Work out the finished part from the listing and answer in its coordinate system (mm). A direction names the side the tool comes from. Round coordinates to 2 decimals unless told otherwise and drop trailing zeros. Order: outer loops, then holes, each group sorted by start corner. A loop starts at its lowest first (then second) coordinate and runs counter-clockwise, first axis right, second up. Notation, with made-up numbers: (34.25, -20) -> (89.25, -20) arc R13 ccw to (89.25, -8) -> close; hole circle Ø3 at (5.25, 62.25). An arc over 180 degrees is marked (long way). Use a Markdown table: item, result. Add a question column.
Item 1: A cutting plane is placed at A-A, the plane z = 5.5. Determine the outline of the cut face in (x, y), plus the area to 3 significant figures.
Item 2: Flat-ended cylindrical pins translate along their axes: P1, Ø10, axis at x = 18, y = 11, coming from the -Z side; P2, Ø4, axis at y = 19.5, z = 12.5, coming from the +X side; P3, Ø1, axis at x = 29.5, z = 3, coming from the -Y side; P4, Ø5, axis at y = 22, z = 13.5, coming from the -X side. Find the tip coordinate at first contact, or state that the pin passes through.
Item 3: A cutting plane is placed at B-B, the plane y = 17.25. Determine the outline of the cut face in (x, z), plus the area to 3 significant figures.
Item 4: Find the intervals of material crossed by L1, parallel to Z at x = 20, y = 11.5; L2, parallel to X at y = 5.5, z = 1.5; L3, parallel to X at y = 12.25, z = 4.5, in increasing order. Write a range as [from, to].
Item 5: A cutting plane is placed at D-D, the plane z = 16. Determine the outline of the cut face in (x, y).
Item 6: For a pull along X with two mould halves and no side action, classify faces 3 (the flat face through (6, 13, 0)), 4 (the flat face through (31.66, 12.52, 12.88)), 5 (the flat face through (12.7, 13, 3)), 6 (the flat face through (19, 13, 6.35)) as +X half, -X half, draft (parallel to the pull), parting line (faces both ways), or undercut.
Item 7: A tool of negligible diameter and unlimited length cuts with its end or side. For faces 1 (the flat face through (19, 25.4, 13)), 2 (the flat face through (25.4, 13, 3)), from which of +Z, -Z, +X, -X, +Y, -Y can it reach the whole face along a straight path? Write none if from no direction.
Item 8: A cutting plane is placed at C-C, the plane x = 4. Determine the outline of the cut face in (y, z), plus the area to 3 significant figures.
from build123d import *

# Parameters (mm, degrees)
F1_DEPTH = 25.4
F3_DEPTH = 25.4


with BuildPart() as f1:
    # F0 (on Front) → F1 (new body)
    with BuildSketch(Plane.XZ):
        Polygon((0, 25.4), (0, 0), (12.7, 0), (12.7, 6.35), (25.4, 6.35), (25.4, 0), (38.1, 0), (38.1, 25.4), align=None)
    extrude(amount=-F1_DEPTH)

    # F2 (on face) → F3 (cut)
    with BuildSketch(Plane.XZ):
        Polygon((0, 25.4), (0, 0), (12.7, 25.4), align=None)
        Polygon((38.1, 25.4), (25.4, 25.4), (38.1, 0), align=None)
    extrude(amount=-F3_DEPTH, mode=Mode.SUBTRACT)


solid = f1.part
Reported:
| question | item | result |
|---|---|---|
| 1 | outline | (2.75, 0) -> (12.7, 0) -> (12.7, 25.4) -> (2.75, 25.4) -> close; (25.4, 0) -> (35.35, 0) -> (35.35, 25.4) -> (25.4, 25.4) -> close |
| 1 | area | 505 mm² |
| 2 | P1 | z = 6.35 |
| 2 | P2 | x = 32.85 |
| 2 | P3 | y = 0 |
| 2 | P4 | x = 5.5 |
| 3 | outline | (0, 0) -> (12.7, 0) -> (12.7, 6.35) -> (25.4, 6.35) -> (25.4, 0) -> (38.1, 0) -> (25.4, 25.4) -> (12.7, 25.4) -> close |
| 3 | area | 565 mm² |
| 4 | L1 | [6.35, 25.4] |
| 4 | L2 | [0.75, 12.7], [25.4, 37.35] |
| 4 | L3 | [2.25, 12.7], [25.4, 35.85] |
| 5 | outline | (8, 0) -> (30.1, 0) -> (30.1, 25.4) -> (8, 25.4) -> close |
| 6 | face 3 | draft |
| 6 | face 4 | +X half |
| 6 | face 5 | undercut |
| 6 | face 6 | undercut |
| 7 | face 1 | +Z, -Z, +X, -X, +Y |
| 7 | face 2 | -Z, +Y, -Y |
| 8 | outline | (0, 0) -> (25.4, 0) -> (25.4, 8) -> (0, 8) -> close |
| 8 | area | 203 mm² |
